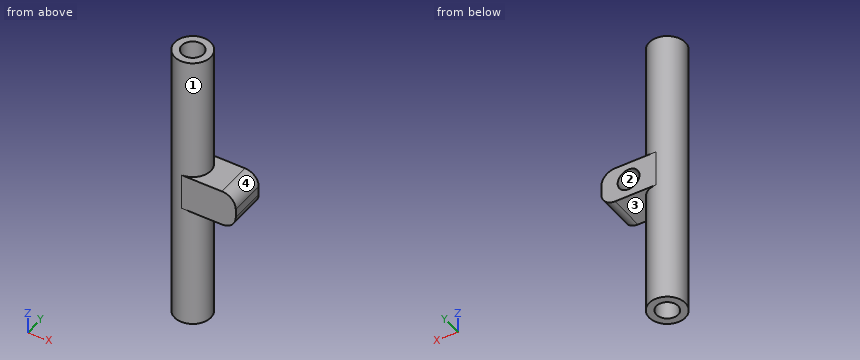
from build123d import *

# Parameters (mm, degrees)
SKETCH1_R           = 15.875
SKETCH1_R_2         = 9.525
BOSS_EXTRUDE1_DEPTH = 125
BOSS_EXTRUDE2_DEPTH = 15.875
SKETCH2_R           = 9.525
CUT_EXTRUDE1_DEPTH  = 25.4
FILLET1_R           = 12


with BuildPart() as part:
    # Sketch1 → Boss-Extrude1 (new body, symmetric)
    with BuildSketch(Plane.XY):
        Circle(SKETCH1_R)
        Circle(SKETCH1_R_2, mode=Mode.SUBTRACT)
    extrude(amount=BOSS_EXTRUDE1_DEPTH, both=True)

    # Sketch1_3 → Boss-Extrude2 (add, symmetric)
    with BuildSketch(Plane.XY):
        with BuildLine():
            Line((0, -15.875), (47.625, -15.875))
            Line((47.625, -15.875), (47.625, 15.875))
            Line((47.625, 15.875), (0, 15.875))
            ThreePointArc((0, 15.875), (11.225320151, 11.225320151), (15.875, 0))
            ThreePointArc((15.875, 0), (11.225320151, -11.225320151), (0, -15.875))
        make_face()
    extrude(amount=BOSS_EXTRUDE2_DEPTH, both=True)

    # Sketch2 → Cut-Extrude1 (cut)
    with BuildSketch(Plane(origin=(0, 15.875, 0), x_dir=(1, 0, 0), z_dir=(0, 1, 0))):
        with Locations((23.8125, 0)):
            Circle(SKETCH2_R)
    extrude(amount=-CUT_EXTRUDE1_DEPTH, mode=Mode.SUBTRACT)

    # Fillet1
    fillet1_edges = [part.edges().sort_by_distance(p)[0] for p in [
        (47.625, 0, -15.875),
        (47.625, 0, 15.875),
    ]]
    fillet(fillet1_edges, radius=FILLET1_R)


solid = part.part
Geometry: final body of the model. Coordinates: model frame, mm. Face numbers are marked on the shaded views. Give positions to 0.01 mm unless a question says otherwise; leave off trailing zeros. Write each loop counter-clockwise with the first axis right and the second up, starting at its lowest first coordinate (ties: lowest second). Pieces come first, ordered by that corner, then holes. Notation, with made-up numbers: (44.25, 48.5) -> (80.25, 48.5) arc R8 cw to (80.25, 60.5) -> close; hole circle Ø6 at (73.5, 37). An arc over 180 degrees is marked (long way). Answer in a Markdown table with one row per item.
(1) Draft query along Z for the marked faces 1, 2, 3 and 4. Return one class per face: +Z half, -Z half, draft (parallel to the pull), parting line (faces both ways), or undercut.
Answers below:
| item | result |
|---|---|
| face 1 | draft |
| face 2 | undercut |
| face 3 | -Z half |
| face 4 | +Z half |
(2) Section query D-D on x = 19.5. Return loops of the section in (y, z) (3 decimals), then the cut area to 3 significant figures.
Answers below:
| item | result |
|---|---|
| outline | (-15.875, -15.875) -> (15.875, -15.875) -> (15.875, -8.493) -> (-9.525, -8.493) -> (-9.525, 8.493) -> (15.875, 8.493) -> (15.875, 15.875) -> (-15.875, 15.875) -> close |
| area | 577 mm^2 |
(3) Section query C-C on x = -6.5. Return loops of the section in (y, z), then the cut area to 3 significant figures.
Answers below:
| item | result |
|---|---|
| outline | (-14.48, -125) -> (-6.96, -125) -> (-6.96, 125) -> (-14.48, 125) -> close; (6.96, -125) -> (14.48, -125) -> (14.48, 125) -> (6.96, 125) -> close |
| area | 3,760 mm^2 |
(4) Section query A-A on y = 7. State how many separate pieces and enclosed holes the cut face has, then the cut area to 3 significant figures.
Answers below:
| item | result |
|---|---|
| separate pieces | 2 |
| enclosed holes | 1 |
| area | 4,610 mm^2 |
(5) Ray query, line 1 along X through (y, z) = (3.25, 0) (1 decimal); line 2 along X through (y, z) = (3, 0) (1 decimal); line 3 along Y through (x, z) = (0, -47) (3 decimals). Return the intervals inside material, ascending. Write a range as [from, to].
Answers below:
| item | result |
|---|---|
| line 1 | [-15.5, -9], [9, 14.3], [33.3, 47.6] |
| line 2 | [-15.6, -9], [9, 14.3], [33.3, 47.6] |
| line 3 | [-15.875, -9.525], [9.525, 15.875] |
(6) Pin query (flat end, axial travel): pin 1 (6 mm diameter, centred on y = 6, z = 75, fed in from +X); pin 2 (5 mm diameter, centred on y = 7, z = -96, fed in from +X); pin 3 (12 mm diameter, centred on y = -9.5, z = 38.5, fed in from -X). Return the tip coordinate at first contact, or that it passes through.
Answers below:
| item | result |
|---|---|
| pin 1 | x = 15.59 |
| pin 2 | x = 15.22 |
| pin 3 | x = -15.48 |
